from build123d import *

# Parameters (mm, degrees)
SKETCH_1_R          = 45
EXTRUDE_1_DEPTH     = 7
SKETCH_2_R          = 25
EXTRUDE_2_DEPTH     = 70
FILLET_1_R          = 3
SKETCH_3_R          = 2.5
CUT_EXTRUDE_3_DEPTH = 35
SKETCH_5_R          = 2.5
CUT_EXTRUDE_4_DEPTH = 35
SKETCH_6_R          = 12.5
CUT_EXTRUDE_5_DEPTH = 36
SKETCH_7_W          = 10.064755008
SKETCH_7_H          = 68.890859038
SKETCH_7_W_2        = 9.000001362
SKETCH_7_H_2        = 72.567998157
CUT_EXTRUDE_6_DEPTH = 35
SKETCH_9_W          = 74.471064375
SKETCH_9_H          = 8.374114708
CUT_EXTRUDE_8_DEPTH = 35
SKETCH_10_R         = 5
CUT_EXTRUDE_1_DEPTH = 110.684759554
CHAMFER_1_SIZE      = 8
CHAMFER_1_SIZE2     = 21.979819356


with BuildPart() as part:
    # Эскиз1 → Вытянуть1 (new body)
    with BuildSketch(Plane.XY):
        Circle(SKETCH_1_R)
    extrude(amount=EXTRUDE_1_DEPTH)

    # Эскиз2 → Вытянуть2 (add)
    with BuildSketch(Plane.XY.offset(7)):
        Circle(SKETCH_2_R)
    extrude(amount=EXTRUDE_2_DEPTH)

    # Скругление1
    fillet_1_edges = [part.edges().sort_by_distance(p)[0] for p in [
        (-25, 0, 77),
    ]]
    fillet(fillet_1_edges, radius=FILLET_1_R)

    # Эскиз3 → Вытянуть3 (cut, symmetric)
    with BuildSketch(Plane(origin=(0, 0, 0), x_dir=(1, 0, 0), z_dir=(0, 1, 0))):
        with Locations(Location((0, -12, 0), (0, 0, 270))):
            Circle(SKETCH_3_R)
        with Locations(Location((0, -25, 0), (0, 0, 270))):
            Circle(SKETCH_3_R)
    extrude(amount=CUT_EXTRUDE_3_DEPTH, both=True, mode=Mode.SUBTRACT)

    # Эскиз5 → Вытянуть4 (cut, symmetric)
    with BuildSketch(Plane(origin=(0, 0, 0), x_dir=(0, 0, -1), z_dir=(1, 0, 0))):
        with Locations((-12, 0)):
            Circle(SKETCH_5_R)
        with Locations((-25, 0)):
            Circle(SKETCH_5_R)
    extrude(amount=CUT_EXTRUDE_4_DEPTH, both=True, mode=Mode.SUBTRACT)

    # Эскиз6 → Вытянуть5 (cut)
    with BuildSketch(Plane(origin=(0, 0, 0), x_dir=(-1, 0, 0), z_dir=(0, 0, -1))):
        Circle(SKETCH_6_R)
    extrude(amount=-CUT_EXTRUDE_5_DEPTH, mode=Mode.SUBTRACT)

    # Эскиз7 → Вытянуть6 (cut, symmetric)
    with BuildSketch(Plane(origin=(0, 0, 0), x_dir=(1, 0, 0), z_dir=(0, 1, 0))):
        with Locations((0, -74)):
            Rectangle(SKETCH_7_W, SKETCH_7_H)
        with Locations((23.349405244, -43.283999079)):
            Rectangle(SKETCH_7_W_2, SKETCH_7_H_2)
        with Locations((-23.349405244, -43.283999079)):
            Rectangle(SKETCH_7_W_2, SKETCH_7_H_2)
    extrude(amount=CUT_EXTRUDE_6_DEPTH, both=True, mode=Mode.SUBTRACT)

    # Эскиз9 → Вытянуть8 (cut, symmetric)
    with BuildSketch(Plane(origin=(0, 0, 0), x_dir=(0, 0, -1), z_dir=(1, 0, 0))):
        with Locations((-44.235532188, 28.187057354)):
            Rectangle(SKETCH_9_W, SKETCH_9_H)
        with Locations((-44.235532188, -28.187057354)):
            Rectangle(SKETCH_9_W, SKETCH_9_H)
    extrude(amount=CUT_EXTRUDE_8_DEPTH, both=True, mode=Mode.SUBTRACT)

    # Эскиз10 → Вырез-Вытянуть1 (cut, through all)
    with BuildSketch(Plane.ZY.offset(18.849404563)):
        with Locations((58.486255415, 0)):
            Circle(SKETCH_10_R)
    extrude(amount=-CUT_EXTRUDE_1_DEPTH, mode=Mode.SUBTRACT)

    # Фаска1
    chamfer_1_edges = [part.edges().sort_by_distance(p)[0] for p in [
        (0, 24, 39.554570481),
    ]]
    chamfer_1_side = [part.faces().sort_by_distance(p)[0] for p in [
        (0, 24, 32.18588004),
    ]]
    chamfer(chamfer_1_edges, length=CHAMFER_1_SIZE, length2=CHAMFER_1_SIZE2, reference=chamfer_1_side[0])


solid = part.part
The listing builds one solid part. Answer for the finished solid, in the listing's coordinates (mm). A direction names the side the tool comes from. Round coordinates to 2 decimals unless told otherwise and drop trailing zeros. Write each loop counter-clockwise with the first axis right and the second up, starting at its lowest first coordinate (ties: lowest second). Pieces come first, ordered by that corner, then holes. Notation, with made-up numbers: M -27.5,-15.5 L -15.5,-15.5 A25 ccw -15.5,-3.5 Z; hole C 75,68 d5. An arc over 180 degrees is marked long. Write each question's results on one line, items separated by ' | '. Start each with the question number.
Item 1: Find section D-D on y = 9. Write down the section's boundary in (x, z).
Item 2: The mould has two halves that part along Z. Classify faces 1 (the flat face through (19, 1, 7)), 2 (the cylindrical face through (13.55, 21.01, 40.03)), 3 (the cylindrical face through (15.6, 0.1, 27.5)): +Z half, -Z half, draft (parallel to the pull), parting line (faces both ways), or undercut.
Item 3: Which of the six approach directions +Z, -Z, +X, -X, +Y, -Y give full straight-line access (tool end or side, diameter ignored) to faces 4 (the cylindrical face through (-13.38, 21.12, 40.03)), 5 (the cylindrical face through (-13.55, -21.01, 40.03)), 6 (the cylindrical face through (13.38, -21.12, 40.03))?
Item 4: Find section C-C on z = 33. Write down the section's boundary in (x, y), and give its area (3 significant figures).
Item 5: Straight lines are drawn through the part: probe 1 along X at (y, z) = (16, 12); probe 2 along Z at (x, y) = (-33, -12); probe 3 along X at (y, z) = (-19, 25). For each, find the intervals that lie inside material, in ascending order.
Item 6: Given pin 1 Ø3 at (y, z) = (0, 25) entering from -X; pin 2 Ø10 at (x, z) = (-23.5, 51.5) entering from +Y; pin 3 Ø1.5 at (x, z) = (3, 9.5) entering from -Y; pin 4 Ø3 at (x, y) = (3, 26) entering from +Z, each flat-ended and moving along its own axis, determine where each tip first touches the part or whether it passes through.
Item 7: Find section A-A on z = 25. Write down the section's boundary in (x, y).
Answer block:
1) outline: M -44.09,0 L -8.67,0 L -8.67,36 L 8.67,36 L 8.67,0 L 44.09,0 L 44.09,7 L 18.85,7 L 18.85,77 L 5.03,77 L 5.03,37.01 L -5.03,37.01 L -5.03,77 L -18.85,77 L -18.85,7 L -44.09,7 Z
2) face 1: +Z half | face 2: draft | face 3: undercut
3) face 4: +Z, -X, +Y | face 5: +Z, -X, -Y | face 6: +Z, +X, -Y
4) outline: M -18.85,-16.42 A25 ccw -7,-24 L 7,-24 A25 ccw 18.85,-16.42 L 18.85,16.42 A25 ccw 7,24 L 5.03,24 L 5.03,20.03 L -5.03,20.03 L -5.03,24 L -7,24 A25 ccw -18.85,16.42 Z; hole C 0,0 d25 | area: 1,140 mm²
5) probe 1: x = -18.85 to -2.5, 2.5 to 18.85 | probe 2: z = 0 to 7 | probe 3: x = -16.25 to -2.5, 2.5 to 16.25
6) pin 1: passes through | pin 2: stops at y = 16.82 | pin 3: stops at y = -24 | pin 4: stops at z = 7
7) outline: M -18.85,-16.42 A25 ccw -7,-24 L -2.5,-24 L -2.5,-12.25 A12.5 cw -12.25,-2.5 L -18.85,-2.5 Z; M -18.85,2.5 L -12.25,2.5 A12.5 cw -2.5,12.25 L -2.5,24 L -7,24 A25 ccw -18.85,16.42 Z; M 2.5,-24 L 7,-24 A25 ccw 18.85,-16.42 L 18.85,-2.5 L 12.25,-2.5 A12.5 cw 2.5,-12.25 Z; M 2.5,12.25 A12.5 cw 12.25,2.5 L 18.85,2.5 L 18.85,16.42 A25 ccw 7,24 L 2.5,24 Z
